from build123d import *

# Parameters (mm, degrees)
MODEL_R             = 2.1
BOSS_EXTRUDE1_DEPTH = 3.125


with BuildPart() as part:
    # Model → Boss-Extrude1 (new body)
    with BuildSketch(Plane.XY):
        with BuildLine():
            Line((175.590993043, 0), (192.911501119, 10))
            Line((192.911501119, 10), (148.776258635, 86.444482386))
            Line((148.776258635, 86.444482386), (131.455750559, 76.444482386))
            Line((131.455750559, 76.444482386), (61.455750559, 76.444482386))
            Line((61.455750559, 76.444482386), (44.135242484, 86.444482386))
            Line((44.135242484, 86.444482386), (0, 10))
            Line((0, 10), (17.320508076, 0))
            ThreePointArc((17.320508076, 0), (96.455750559, 15.314685), (175.590993043, 0))
        make_face()
        with Locations((42.795496522, 64.123974311)):
            Circle(MODEL_R, mode=Mode.SUBTRACT)
        with Locations((18.660254038, 22.320508076)):
            Circle(MODEL_R, mode=Mode.SUBTRACT)
        with Locations((150.116004597, 64.123974311)):
            Circle(MODEL_R, mode=Mode.SUBTRACT)
        with Locations((174.251247081, 22.320508076)):
            Circle(MODEL_R, mode=Mode.SUBTRACT)
        with BuildLine():
            Line((54.855750559, 29.174833766), (54.855750559, 19.174833766))
            ThreePointArc((54.855750559, 19.174833766), (53.255750559, 17.574833766), (51.655750559, 19.174833766))
            Line((51.655750559, 19.174833766), (51.655750559, 29.174833766))
            ThreePointArc((51.655750559, 29.174833766), (53.255750559, 30.774833766), (54.855750559, 29.174833766))
        make_face(mode=Mode.SUBTRACT)
        with BuildLine():
            Line((141.255750559, 29.174833766), (141.255750559, 19.174833766))
            ThreePointArc((141.255750559, 19.174833766), (139.655750559, 17.574833766), (138.055750559, 19.174833766))
            Line((138.055750559, 19.174833766), (138.055750559, 29.174833766))
            ThreePointArc((138.055750559, 29.174833766), (139.655750559, 30.774833766), (141.255750559, 29.174833766))
        make_face(mode=Mode.SUBTRACT)
    extrude(amount=BOSS_EXTRUDE1_DEPTH)


solid = part.part
For this review, take the finished solid that the model builds, in its own axes (mm). A direction names the side the tool comes from. Round coordinates to 2 decimals unless told otherwise and drop trailing zeros. Write each loop counter-clockwise with the first axis right and the second up, starting at its lowest first coordinate (ties: lowest second). Pieces come first, ordered by that corner, then holes. Notation, with made-up numbers: (-29, -40) - (14, -40) arc R9 ccw to (14, -28) - close; hole circle Ø1 at (72.5, 34). An arc over 180 degrees is marked (long way). Use a Markdown table: item, result.
Q1. The part is to be moulded in two halves that separate along X. For faces 3 (the flat face through (184.13, 4.93, 1.54)), 4 (the flat face through (52.917, 81.374, 1.541)), 5 (the flat face through (95, 44, 0)), 6 (the cylindrical face through (176.191, 21.516, 1.541)), say which applies: pulls with the +X half, pulls with the -X half, needs draft (parallel to the pull), parting line crosses it, or undercut.
Derived:
| item | result |
|---|---|
| face 3 | pulls with the +X half |
| face 4 | undercut |
| face 5 | needs draft |
| face 6 | undercut |
Q2. Machinability: for faces 1 (the flat face through (22.4, 48.8, 1.5)), 2 (the flat face through (140.237, 81.514, 1.541)), which of the approach directions +Z, -Z, +X, -X, +Y, -Y give a long, thin tool a straight path to every point of the face, cutting with its end or side? Answer none if there is none.
Derived:
| item | result |
|---|---|
| face 1 | +Z, -Z, -X, +Y |
| face 2 | +Z, -Z, +Y |
Q3. We need section C-C (x = 79.5). Give the boundary of the cut face in (y, z) (3 decimals).
Derived:
| item | result |
|---|---|
| outline | (14.636, 0) - (76.444, 0) - (76.444, 3.125) - (14.636, 3.125) - close |
Q4. Clearance check with flat-ended pins moving along their axes: pin 1 (0.9 mm diameter, centred on x = 98, z = 1, fed in from +Y); pin 2 (4 mm diameter, centred on x = 18.66, y = 22.32, fed in from +Z); pin 3 (0.9 mm diameter, centred on y = 22.5, z = 2, fed in from +X). State where each tip first meets the part, or that it passes through.
Derived:
| item | result |
|---|---|
| pin 1 | stops at y = 76.44 |
| pin 2 | passes through |
| pin 3 | stops at x = 185.95 |
Q5. We need section B-B (y = 47.5). Give the boundary of the cut face in (x, z) (3 decimals).
Derived:
| item | result |
|---|---|
| outline | (21.651, 0) - (171.261, 0) - (171.261, 3.125) - (21.651, 3.125) - close |
Q6. Wall thickness on line 1 along X through (y, z) = (22.5, 1.6); line 2 along X through (y, z) = (27, 0.25); line 3 along Y through (x, z) = (99.5, 1.9): over which ranges is each line inside the solid? List them lowest first.
Derived:
| item | result |
|---|---|
| line 1 | x = 7.22 to 16.57, 20.75 to 51.66, 54.86 to 138.06, 141.26 to 172.16, 176.34 to 185.69 |
| line 2 | x = 9.81 to 51.66, 54.86 to 138.06, 141.26 to 183.1 |
| line 3 | y = 15.29 to 76.44 |
Q7. We need section A-A (z = 1.7). Give the boundary of the cut face in (x, y).
Derived:
| item | result |
|---|---|
| outline | (0, 10) - (17.32, 0) arc R212.11 cw to (175.59, 0) - (192.91, 10) - (148.78, 86.44) - (131.46, 76.44) - (61.46, 76.44) - (44.14, 86.44) - close; hole circle Ø4.2 at (18.66, 22.32); hole circle Ø4.2 at (42.8, 64.12); hole (51.66, 19.17) arc R1.6 ccw to (54.86, 19.17) - (54.86, 29.17) arc R1.6 ccw to (51.66, 29.17) - close; hole (138.06, 19.17) arc R1.6 ccw to (141.26, 19.17) - (141.26, 29.17) arc R1.6 ccw to (138.06, 29.17) - close; hole circle Ø4.2 at (150.12, 64.12); hole circle Ø4.2 at (174.25, 22.32) |
